Source: CAD feature listing. Evaluate the final solid. Frame: model axes, mm. Face numbers are marked on the shaded views. A direction names the side the tool comes from. Give positions to 0.01 mm unless a question says otherwise; leave off trailing zeros. Loops run counter-clockwise (first coordinate to the right, second up) from the corner with the lowest first, then second, coordinate; pieces in that order, holes last. Notation, with made-up numbers: M 77.25,-9.75 L 86.25,-9.75 A27 cw 86.25,11.25 Z; hole C -16.75,-5 d8. An arc over 180 degrees is marked long. Put each result on its own line as item: value.
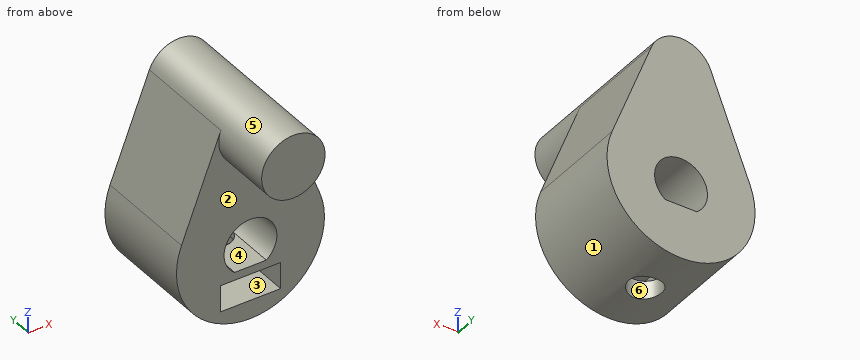
from build123d import *

# Parameters (mm, degrees)
SKETCH1_R                = 7
BOSS_EXTRUDE1_DEPTH      = 10
SKETCH3_W                = 5.7
SKETCH3_H                = 2.5
CUT_EXTRUDE1_DEPTH       = 8
SKETCH6_R                = 1.55
CUT_EXTRUDE2_DEPTH       = 15.071247279
BOSS_EXTRUDE2_DEPTH      = 6
BOSS_EXTRUDE2_DEPTH_BACK = 10
SKETCH7_R                = 3
BOSS_EXTRUDE3_START      = -10
BOSS_EXTRUDE3_DEPTH      = 10


with BuildPart() as part:
    # Sketch1 → Boss-Extrude1 (new body)
    with BuildSketch(Plane(origin=(0, 0, 0), x_dir=(1, 0, 0), z_dir=(0, 1, 0))):
        with Locations(Location((0, 0, 0), (0, 0, 270))):
            Circle(SKETCH1_R)
        with BuildLine():
            Line((-1.5, 2), (1.5, 2))
            ThreePointArc((1.5, 2), (0, -2.5), (-1.5, 2))
        make_face(mode=Mode.SUBTRACT)
    extrude(amount=BOSS_EXTRUDE1_DEPTH)

    # Sketch3 → Cut-Extrude1 (cut)
    with BuildSketch(Plane(origin=(0, 0, 0), x_dir=(1, 0, 0), z_dir=(0, 1, 0))):
        with Locations((0, 4)):
            Rectangle(SKETCH3_W, SKETCH3_H)
    extrude(amount=CUT_EXTRUDE1_DEPTH, mode=Mode.SUBTRACT)

    # Sketch6 → Cut-Extrude2 (cut, through all)
    with BuildSketch(Plane.XY):
        with Locations(Location((0, 5, 0), (0, 0, 345.407449398))):
            Circle(SKETCH6_R)
    extrude(amount=-CUT_EXTRUDE2_DEPTH, mode=Mode.SUBTRACT)



with BuildPart() as body_2:
    # Sketch7 → Boss-Extrude2 (new, two sides: drawn at the far end of the back side and taken through both)
    with BuildSketch(Plane.XZ.offset(-BOSS_EXTRUDE2_DEPTH_BACK)):
        with Locations(Location((0, 11, 0), (0, 0, 270))):
            Circle(SKETCH7_R)
    extrude(amount=BOSS_EXTRUDE2_DEPTH + BOSS_EXTRUDE2_DEPTH_BACK)


with BuildPart() as part_1:
    add(part.part)

    add(body_2.part)  # Boss-Extrude3 merges body 2
    # Sketch9 → Boss-Extrude3 (add)
    with BuildSketch(Plane(origin=(0, 10, 0), x_dir=(1, 0, 0), z_dir=(0, 1, 0)).offset(BOSS_EXTRUDE3_START)):
        with BuildLine():
            ThreePointArc((6.520786851, -2.545454545), (0, -7), (-6.520786851, -2.545454545))
            Line((-6.520786851, -2.545454545), (-2.794622936, -12.090909091))
            ThreePointArc((-2.794622936, -12.090909091), (-0.555036572, -8.051791323), (3, -11))
            ThreePointArc((3, -11), (2.948208677, -11.555036572), (2.794622936, -12.090909091))
            Line((2.794622936, -12.090909091), (6.520786851, -2.545454545))
        make_face()
    extrude(amount=BOSS_EXTRUDE3_DEPTH)


solid = part_1.part
1. Section query B-B (x = 0). Output: boundary loops of the cut face in (y, z).
Found:
outline: M -6,8 L 0,8 L 0,2.5 L 10,2.5 L 10,14 L -6,14 Z; M 0,-7 L 3.45,-7 L 3.45,-5.25 L 0,-5.25 Z; M 0,-2.75 L 3.45,-2.75 L 3.45,-2 L 0,-2 Z; M 6.55,-7 L 10,-7 L 10,-2 L 6.55,-2 L 6.55,-2.75 L 8,-2.75 L 8,-5.25 L 6.55,-5.25 Z
2. Draft query along Z for the marked faces 1, 2 and 3. Return one class per face: pulls with the +Z half, pulls with the -Z half, needs draft (parallel to the pull), parting line crosses it, or undercut.
Found:
face 1: parting line crosses it
face 2: needs draft
face 3: undercut
3. Section query C-C (y = 1.5). Output: boundary loops of the cut face in (x, z).
Found:
outline: M -6.52,2.55 A7 ccw long 6.52,2.55 L 2.79,12.09 A3 ccw -2.79,12.09 Z; hole M -2.85,-5.25 L 2.85,-5.25 L 2.85,-2.75 L -2.85,-2.75 Z; hole M -1.5,-2 L 1.5,-2 A2.5 ccw long Z
4. Material intervals for line 1 (Z direction, x = 0, y = 2.25); line 2 (X direction, y = 4, z = 0); line 3 (Y direction, x = 0, z = -6.6), sorted ascending. Write a range as from..to.
Found:
line 1: -7..-5.25, -2.75..-2, 2.5..14
line 2: -7..-2.5, 2.5..7
line 3: 0..3.45, 6.55..10
5. Section query A-A (z = 0). Output: boundary loops of the cut face in (x, y).
Found:
outline: M -7,0 L -2.5,0 L -2.5,10 L -7,10 Z; M 2.5,0 L 7,0 L 7,10 L 2.5,10 Z
6. Contact query for flat-ended pins moving along their axis: P1, Ø3, axis at x = -4.5, y = 2.5, coming from the -Z side; P2, Ø4, axis at y = 7.5, z = 4.5, coming from the -X side; P3, Ø1.2, axis at y = 4.5, z = -4, coming from the +X side; P4, Ø1.7, axis at x = -0.5, y = 3, coming from the +Z side. Output: stop coordinate, or through.
Found:
P1: z = -6.32
P2: x = -6.54
P3: x = 6.12
P4: z = 14
7. Access query for the marked faces 4, 5 and 6. Directions: +Z, -Z, +X, -X, +Y, -Y. A direction counts if a zero-diameter tool reaches every point of the face in a straight line with its end or side. Return the directions, or none.
Found:
face 4: +Y, -Y
face 5: -Y
face 6: -Z
8. Section query D-D (z = 11). Output: boundary loops of the cut face in (x, y), plus the area to 3 significant figures.
Found:
outline: M -3.22,0 L -3,0 L -3,-6 L 3,-6 L 3,0 L 3.22,0 L 3.22,10 L -3.22,10 Z
area: 100 mm^2
